Read the model definition and answer for the solid it produces. Units are mm, in the model's axes. Face numbers are marked on the shaded views. A direction names the side the tool comes from. Coordinates: 2 decimals unless noted, no trailing zeros. Write each loop counter-clockwise with the first axis right and the second up, starting at its lowest first coordinate (ties: lowest second). Pieces come first, ordered by that corner, then holes.
(1) Determine the mould class of the marked faces 3, 4 and 5 for opening direction X: pulls with the +X half, pulls with the -X half, needs draft (parallel to the pull), parting line crosses it, or undercut.
(2) Straight lines are drawn through the part: line 1 along X through (y, z) = (0, 19.5); line 2 along Y through (x, z) = (16, 1); line 3 along Y through (x, z) = (0, 3). For each, find the intervals that lie inside material, in ascending order.
(3) Which of the six approach directions +Z, -Z, +X, -X, +Y, -Y give full straight-line access (tool end or side, diameter ignored) to the marked faces 1 and 2?
(4) The part is cut by section B-B, the plane y = 16.5. Determine the outline of the cut face in (x, z), and give its area (3 significant figures).
(5) Given pin 1 (4 mm diameter, centred on x = 16.1, y = -9.51, fed in from +Z); pin 2 (10 mm diameter, centred on x = -12, y = 11, fed in from -Z); pin 3 (3 mm diameter, centred on x = -23, z = 25, fed in from -Y), each flat-ended and moving along its own axis, determine where each tip first touches the part or whether it passes through.
(6) The part is cut by section C-C, the plane z = 3. State how many separate pieces and enclosed holes the cut face has, and give its area (3 significant figures).
```python
from build123d import *

# Parameters (mm, degrees)
SKETCH_W        = 40.7
SKETCH_H        = 47
PAD_DEPTH       = 5
SKETCH001_R     = 18.5
POCKET_DEPTH    = 5.001
SKETCH002_R     = 1.5
POCKET001_DEPTH = 5.001
SKETCH003_W     = 40.7
SKETCH003_H     = 5
PAD001_DEPTH    = 30
SKETCH004_R     = 1.5
POCKET002_DEPTH = 5
PAD002_DEPTH    = 4
PAD003_DEPTH    = 4
SKETCH007_W     = 42
SKETCH007_H     = 44.033375
POCKET003_DEPTH = 32
FILLET_R        = 1


with BuildPart() as part:
    # Sketch → Pad (new body)
    with BuildSketch(Plane.XY):
        with Locations((0, 3.341403)):
            Rectangle(SKETCH_W, SKETCH_H)
    extrude(amount=PAD_DEPTH)

    # Sketch001 → Pocket (cut, through all)
    with BuildSketch(Plane.XY.offset(5)):
        with Locations((0, 6.2129)):
            Circle(SKETCH001_R)
    extrude(amount=-POCKET_DEPTH, mode=Mode.SUBTRACT)

    # Sketch002 → Pocket001 (cut, through all)
    with BuildSketch(Plane.XY.offset(5)):
        with Locations((-16.1, 22.6911)):
            Circle(SKETCH002_R)
        with Locations((16.1, 22.6911)):
            Circle(SKETCH002_R)
        with Locations((16.1, -9.5089)):
            Circle(SKETCH002_R)
        with Locations((-16.1, -9.5089)):
            Circle(SKETCH002_R)
    extrude(amount=-POCKET001_DEPTH, mode=Mode.SUBTRACT)

    # Sketch003 → Pad001 (new body)
    with BuildSketch(Plane.XY.offset(5)):
        with Locations((0, -17.674198)):
            Rectangle(SKETCH003_W, SKETCH003_H)
    extrude(amount=PAD001_DEPTH)

    # Sketch004 → Pocket002 (cut)
    with BuildSketch(Plane(origin=(0, -15.174198, 0), x_dir=(-1, 0, 0), z_dir=(0, 1, 0))):
        with Locations((9.963108, 10.997544)):
            Circle(SKETCH004_R)
        with Locations((-16.42986, 29.9825)):
            Circle(SKETCH004_R)
        with Locations((16.42986, 29.9825)):
            Circle(SKETCH004_R)
    extrude(amount=-POCKET002_DEPTH, mode=Mode.SUBTRACT)

    # Sketch005 → Pad002 (new body)
    with BuildSketch(Plane.YZ.offset(20.35)):
        Polygon((-20.1666, 0), (26.8334, 0), (26.8334, 5), (-15.1666, 35), (-20.1666, 35), align=None)
    extrude(amount=PAD002_DEPTH)

    # Sketch006 → Pad003 (new body)
    with BuildSketch(Plane(origin=(-20.35, 0, 0), x_dir=(0, -1, 0), z_dir=(-1, 0, 0))):
        Polygon((-26.8425, 0), (20.1575, 0), (20.1575, 35), (15.1575, 35), (-26.8425, 5), align=None)
    extrude(amount=PAD003_DEPTH)

    # Sketch007 → Pocket003 (cut)
    with BuildSketch(Plane.XY.offset(5)):
        with Locations((0, 6.547751)):
            Rectangle(SKETCH007_W, SKETCH007_H)
    extrude(amount=POCKET003_DEPTH, mode=Mode.SUBTRACT)

    # Fillet
    fillet_edges = [part.edges().sort_by_distance(p)[0] for p in [
        (-24.35, 26.8425, 2.5),
        (24.35, 26.8334, 2.5),
    ]]
    fillet(fillet_edges, radius=FILLET_R)


solid = part.part
```
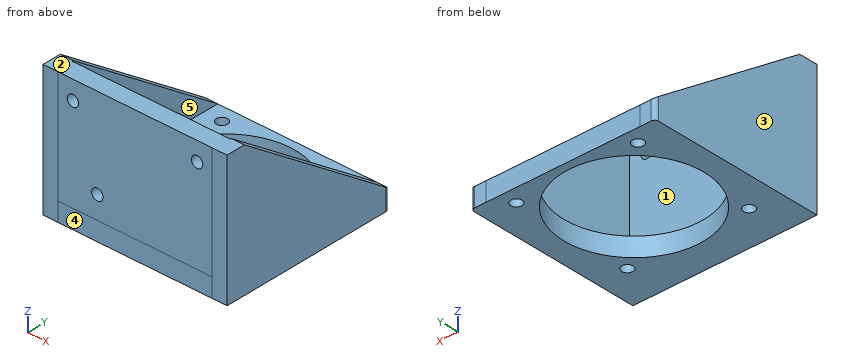
Computed:
1. face 3: pulls with the -X half
1. face 4: needs draft
1. face 5: undercut
2. line 1: x = -24.35 to -21, 21 to 24.35
2. line 2: y = -20.16 to -11.01, -8.01 to -3.07, 15.5 to 21.19, 24.19 to 26.84
2. line 3: y = -20.16 to -12.29, 24.71 to 26.84
3. face 1: +Z, +Y
3. face 2: +Z, +X, -X, +Y, -Y
4. outline: (-24.35, 0) - (-15.38, 0) - (-15.38, 5) - (-21, 5) - (-21, 12.39) - (-24.35, 12.39) - close; (15.38, 0) - (24.35, 0) - (24.35, 12.38) - (21, 12.38) - (21, 5) - (15.38, 5) - close
4. area: 139 mm2
5. pin 1: stops at z = 5
5. pin 2: passes through
5. pin 3: stops at y = -20.16
6. separate pieces: 1
6. enclosed holes: 5
6. area: 1,180 mm2
